For this review, take the finished solid that the model builds, in its own axes (mm). Face numbers are marked on the shaded views. A direction names the side the tool comes from. Coordinates: 2 decimals unless noted, no trailing zeros. Write each loop counter-clockwise with the first axis right and the second up, starting at its lowest first coordinate (ties: lowest second). Pieces come first, ordered by that corner, then holes. Notation, with made-up numbers: (-31.75, -0.75) - (5.25, -0.75) arc R25 ccw to (5.25, 15.25) - close; hole circle Ø2 at (51, 23.5). An arc over 180 degrees is marked (long way). Use one line per item in the form item = value. Start each with the question number.
1) We need section D-D (y = -22). Give the boundary of the cut face in (x, z), plus the area to 3 significant figures.
2) Insertion check: P1, Ø11, axis at x = -8.5, y = -7, coming from the -Z side; P2, Ø24, axis at x = -13.5, z = -4, coming from the +Y side; P3, Ø0.8, axis at x = -13, z = -13, coming from the -Y side. Each pin has a flat end and moves straight along its axis. Give the tip position at first contact, or say it passes through.
3) For L1, parallel to X at y = 4, z = 0; L2, parallel to Y at x = 7, z = -7.5; L3, parallel to X at y = -32, z = 0, list the stretches that pass through material, from the lowest coordinate up. Write a range as from..to.
4) Tool access review of the marked faces 1, 2, 3 and 4: name each direction out of +Z, -Z, +X, -X, +Y, -Y from which nothing blocks a thin tool from reaching the whole face with its end or side.
5) We need section A-A (x = 0). Count the separate pieces of the cut face and the enclosed holes in it, plus the area to 3 significant figures.
6) Mouldability with a two-part tool opening along X and no side actions: class the marked faces 5, 6 and 7 as pulls with the +X half, pulls with the -X half, needs draft (parallel to the pull), parting line crosses it, or undercut.
7) We need section C-C (y = 3.5). Give the boundary of the cut face in (x, z), plus the area to 3 significant figures.
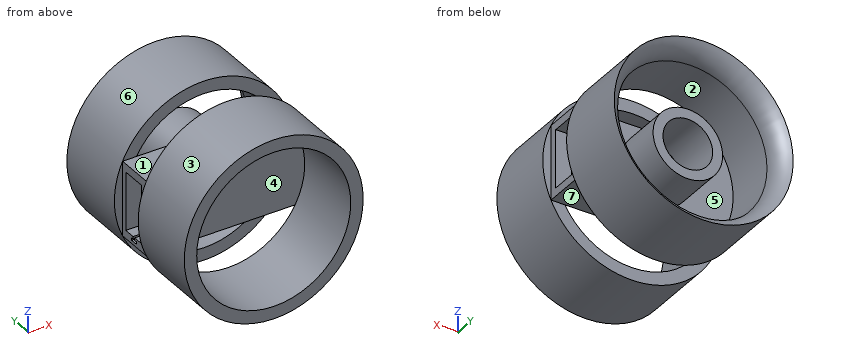
```python
from build123d import *

# Parameters (mm, degrees)
SKETCH_1_R          = 36
EXTRUDE_1_DEPTH     = 30
SKETCH_2_R          = 31
CUT_EXTRUDE_1_DEPTH = 30
FILLET_1_R          = 10
SKETCH_11_W         = 65.4474843869366
SKETCH_11_H         = 30.000000000000004
EXTRUDE_8_DEPTH     = 15
CUT_EXTRUDE_3_DEPTH = 84.18024249227881
CUT_EXTRUDE_4_DEPTH = 58.00000000000003
SKETCH_21_R         = 14
EXTRUDE_10_DEPTH    = 20
SKETCH_22_R         = 10
CUT_EXTRUDE_5_DEPTH = 20
EXTRUDE_START       = 29.000000000000004
SKETCH_23_R         = 36
EXTRUDE_11_DEPTH    = 29.000000000000004
CUT_EXTRUDE_START   = -29
SKETCH_24_R         = 31
CUT_EXTRUDE_7_DEPTH = 29


with BuildPart() as part:
    # 草圖1 → 填料-伸長1 (new body)
    with BuildSketch(Plane(origin=(0, 0, 0), x_dir=(1, 0, 0), z_dir=(0, 1, 0))):
        with Locations(Location((0, 0, 0), (0, 0, 270))):
            Circle(SKETCH_1_R)
    extrude(amount=EXTRUDE_1_DEPTH)

    # 草圖2 → 除料-伸長1 (cut)
    with BuildSketch(Plane(origin=(0, 30, 0), x_dir=(1, 0, 0), z_dir=(0, 1, 0))):
        with Locations(Location((0, 0, 0), (0, 0, 270))):
            Circle(SKETCH_2_R)
    extrude(amount=-CUT_EXTRUDE_1_DEPTH, mode=Mode.SUBTRACT)

    # 圓角1
    # the kernel refuses this fillet: 10 mm, written as the material it takes off along each edge
    with BuildSketch(Plane(origin=(0, 30, 0), x_dir=(-1.8e-16, 0, 1), z_dir=(-1, 0, -1.8e-16))) as fillet_1_piece_1:
        with BuildLine():
            CenterArc((41, -8.660254037844858), FILLET_1_R, 119.99999999999864, 60.000000000001364)
            Line((31.000000000000004, -8.660254037844858), (30.800000000000004, -8.660254037844858))
            Line((30.800000000000004, -8.660254037844858), (30.8, 0))
            Line((30.8, 0), (31, 0.1999999999999993))
            ThreePointArc((31, 0.1999999999999993), (33.5000000000001, 0.1999999999999993), (35.90000000000021, 0.17320508075653507))
            Line((35.90000000000021, 0.17320508075653507), (36.000000000000206, -3.5527e-13))
        make_face()
    revolve(axis=Axis((0, 30, 0), (0, 1, 0)), mode=Mode.SUBTRACT)

    # 草圖11 → 填料-伸長8 (add)
    with BuildSketch(Plane(origin=(0, 0, 0), x_dir=(1, 0, 0), z_dir=(0, 1, 0))):
        Rectangle(SKETCH_11_W, SKETCH_11_H)
    extrude(amount=-EXTRUDE_8_DEPTH)

    # 草圖16 → 除料-伸長3 (cut, through all)
    with BuildSketch(Plane.ZY.offset(32.7237421934683)):
        Polygon((-11.724999999999989, -2.02034535171655), (11.725000000000014, -2.02034535171655), (11.725000000000014, -12.02034535171655), (-11.724999999999985, -12.02034535171655), align=None)
    extrude(amount=-CUT_EXTRUDE_3_DEPTH, mode=Mode.SUBTRACT)

    # 草圖19 → 除料-伸長4 (cut)
    with BuildSketch(Plane.ZY.offset(32.7237421934683)):
        Polygon((-11.72500000000632, -6.624703450403075), (-12.725000000017417, -6.624703450403075), (-12.725000000017417, -5.624703450403075), (-13.725000000017417, -5.624703450403075), (-13.725000000017417, -8.624839762103937), (-12.725000000017417, -8.624839762103937), (-12.725000000017417, -7.624703450403074), (-11.72500000000632, -7.624703450403074), align=None)
    extrude(amount=-CUT_EXTRUDE_4_DEPTH, mode=Mode.SUBTRACT)

    # 草圖21 → 填料-伸長10 (add)
    with BuildSketch(Plane(origin=(0, 0, 0), x_dir=(1, 0, 0), z_dir=(0, 1, 0))):
        with Locations(Location((0, 0, 0), (0, 0, 270))):
            Circle(SKETCH_21_R)
    extrude(amount=EXTRUDE_10_DEPTH)

    # 草圖22 → 除料-伸長5 (cut)
    with BuildSketch(Plane(origin=(0, 20, 0), x_dir=(1, 0, 0), z_dir=(0, 1, 0))):
        with Locations(Location((0, 0, 0), (0, 0, 270))):
            Circle(SKETCH_22_R)
    extrude(amount=-CUT_EXTRUDE_5_DEPTH, mode=Mode.SUBTRACT)

    # 草圖23 → 填料-伸長11 (add)
    with BuildSketch(Plane.XZ.offset(15).offset(EXTRUDE_START)):
        with Locations(Location((0, 0, 0), (0, 0, 90))):
            Circle(SKETCH_23_R)
    extrude(amount=-EXTRUDE_11_DEPTH)

    # 草圖24 → 除料-伸長7 (cut)
    with BuildSketch(Plane.XZ.offset(44.00000000000001).offset(CUT_EXTRUDE_START)):
        with Locations(Location((0, 0, 0), (0, 0, 90))):
            Circle(SKETCH_24_R)
    extrude(amount=CUT_EXTRUDE_7_DEPTH, mode=Mode.SUBTRACT)


solid = part.part
```
Determined:
q1.outline = circle Ø72 at (0, 0); hole circle Ø62 at (0, 0)
q1.area = 1,050 mm²
q2.P1 = -15
q2.P2 = 20
q2.P3 = -15
q3.L1 = -36..-31, -14..-10, 10..14, 31..36
q3.L2 = -15..-12.02, -2.02..20
q3.L3 = -36..-31, 31..36
q4.face_1 = +Z, +X, -X
q4.face_2 = +Y
q4.face_3 = +Y, -Y
q4.face_4 = -Y
q5.separate_pieces = 5
q5.enclosed_holes = 1
q5.area = 936 mm²
q6.face_5 = undercut
q6.face_6 = parting line crosses it
q6.face_7 = needs draft
q7.outline = circle Ø72 at (0, 0); circle Ø28 at (0, 0); hole circle Ø62 at (0, 0); hole circle Ø20 at (0, 0)
q7.area = 1,350 mm²
